Here's how the part is built. I have some questions about the finished solid (model axes, mm). Give positions to 0.01 mm unless a question says otherwise; leave off trailing zeros. Loops run counter-clockwise (first coordinate to the right, second up) from the corner with the lowest first, then second, coordinate; pieces in that order, holes last.
Q1. I'm going to push flat-ended pins straight in: P1, Ø6, axis at y = 8.636, z = -64.897, coming from the +X side; P2, Ø5, axis at x = 4, z = 21, coming from the +Y side; P3, Ø5.5, axis at x = 7.747, z = 83.058, coming from the -Y side; P4, Ø1.4, axis at x = -1, y = 11.5, coming from the -Z side. Where does each tip first touch, or does it pass through?
Q2. I need wall thicknesses on probe 1 along Z at (x, y) = (-0.5, 3); probe 2 along Y at (x, z) = (6.5, 183.5). Which ranges of each line are inside material? Lowest first, please.
Q3. Suppose I cut it at A-A (z = 3.5). List the corners of the cut face in (x, y) for me.
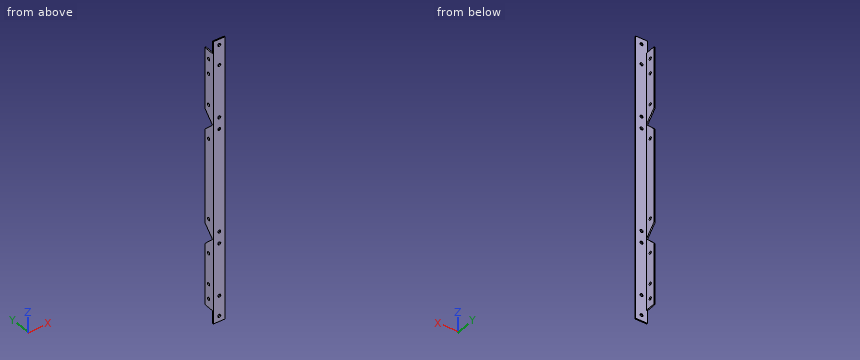
```python
from build123d import *

# Parameters (mm, degrees)
BOSS_EXTRUDE1_DEPTH = 208.28
SKETCH2_R           = 2.38125
CUT_EXTRUDE1_DEPTH  = 1.778
SKETCH3_W           = 19.05
SKETCH3_H           = 1.778
BOSS_EXTRUDE2_DEPTH = 20.32
SKETCH4_R           = 2.38125
CUT_EXTRUDE2_DEPTH  = 1.778


with BuildPart() as part:
    # Sketch1 → Boss-Extrude1 (new body)
    with BuildSketch(Plane.XY):
        Polygon((0, 0), (0, 17.272), (-1.778, 17.272), (-1.778, -1.778), (17.272, -1.778), (17.272, 0), align=None)
    boss_extrude1 = extrude(amount=BOSS_EXTRUDE1_DEPTH)

    # Sketch2 → Cut-Extrude1 (cut)
    with BuildSketch(Plane(origin=(0, 0, 0), x_dir=(0, 0, -1), z_dir=(1, 0, 0))):
        with Locations(Location((-194.31, 8.636, 0), (0, 0, 90))):
            Circle(SKETCH2_R)
        with Locations(Location((-170.434, 8.636, 0), (0, 0, 90))):
            Circle(SKETCH2_R)
        with Locations(Location((-120.269, 8.636, 0), (0, 0, 90))):
            Circle(SKETCH2_R)
        with Locations(Location((-64.897, 8.636, 0), (0, 0, 90))):
            Circle(SKETCH2_R)
        Polygon((-92.583, 0), (-109.855, 17.272), (-75.311, 17.272), align=None)
    cut_extrude1 = extrude(amount=-CUT_EXTRUDE1_DEPTH, mode=Mode.SUBTRACT)

    # Sketch3 → Boss-Extrude2 (add)
    with BuildSketch(Plane.XY.offset(208.28)):
        with Locations((7.747, -0.889)):
            Rectangle(SKETCH3_W, SKETCH3_H)
    boss_extrude2 = extrude(amount=BOSS_EXTRUDE2_DEPTH)

    # Sketch4 → Cut-Extrude2 (cut)
    with BuildSketch(Plane(origin=(0, 0, 0), x_dir=(1, 0, 0), z_dir=(0, 1, 0))):
        with Locations(Location((7.747, -219.456, 0), (0, 0, 180))):
            Circle(SKETCH4_R)
        with Locations(Location((7.747, -83.058, 0), (0, 0, 180))):
            Circle(SKETCH4_R)
        with Locations(Location((7.747, -102.108, 0), (0, 0, 180))):
            Circle(SKETCH4_R)
        with Locations(Location((7.747, -186.944, 0), (0, 0, 180))):
            Circle(SKETCH4_R)
    cut_extrude2 = extrude(amount=-CUT_EXTRUDE2_DEPTH, mode=Mode.SUBTRACT)

    # Mirror3: Boss-Extrude1, Cut-Extrude1, Boss-Extrude2, Cut-Extrude2 across plane
    add(boss_extrude1.mirror(Plane(origin=(0, 0, 0), x_dir=(1, 0, 0), z_dir=(0, 0, -1))))
    add(cut_extrude1.mirror(Plane(origin=(0, 0, 0), x_dir=(1, 0, 0), z_dir=(0, 0, -1))), mode=Mode.SUBTRACT)
    add(boss_extrude2.mirror(Plane(origin=(0, 0, 0), x_dir=(1, 0, 0), z_dir=(0, 0, -1))))
    add(cut_extrude2.mirror(Plane(origin=(0, 0, 0), x_dir=(1, 0, 0), z_dir=(0, 0, -1))), mode=Mode.SUBTRACT)


solid = part.part
```
Solutions:
1. P1: stops at x = 0
1. P2: stops at y = 0
1. P3: stops at y = -1.78
1. P4: stops at z = -208.28
2. probe 1: z = -208.28 to -95.58, -89.58 to 89.58, 95.58 to 208.28
2. probe 2: y = -1.78 to 0
3. outline: (-1.78, -1.78) - (17.27, -1.78) - (17.27, 0) - (0, 0) - (0, 17.27) - (-1.78, 17.27) - close
